Geometry: final body of the model. Coordinates: model frame, mm. Coordinates: 2 decimals unless noted, no trailing zeros. Loops run counter-clockwise (first coordinate to the right, second up) from the corner with the lowest first, then second, coordinate; pieces in that order, holes last. Notation, with made-up numbers: (32, 12.5) - (83, 12.5) arc R24 cw to (83, 41.5) - close; hole circle Ø1 at (8.25, 55). An arc over 180 degrees is marked (long way). Answer in a Markdown table with one row per item.
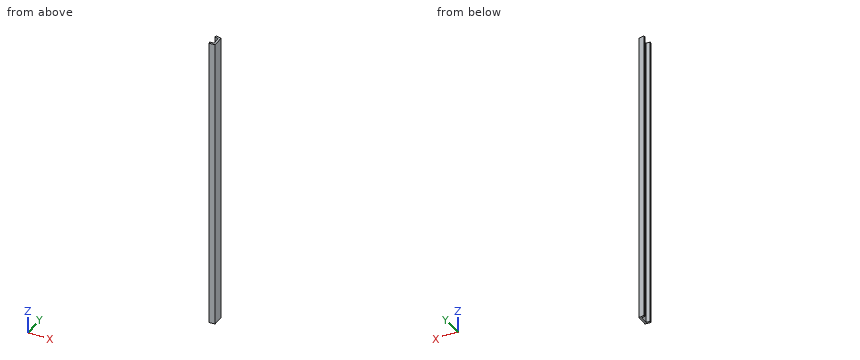
from build123d import *

# Parameters (mm, degrees)
BOSS_EXTRUDE1_DEPTH = 750


with BuildPart() as part:
    # Master sketch-Wing Geometry Master Sketc → Boss-Extrude1 (new body)
    with BuildSketch(Plane.XY):
        with BuildLine():
            Line((224.93, -6.178926254), (224.93, 22.373189537))
            add(Edge.make_bspline(
                [(224.93, 22.373189537), (223.937151031, 22.604229635), (221.53569088, 23.158078559), (217.696277573, 24.019984904), (214.083050592, 24.807059628), (211.880072571, 25.27832033), (211.114806417, 25.441064095)],
                knots=[0.125197771, 0.125197771, 0.125197771, 0.125197771, 0.130088746, 0.137022467, 0.144077656, 0.147831525, 0.147831525, 0.147831525, 0.147831525], degree=3))
            Line((211.114806417, 25.441064095), (210.07475011, 20.55043194))
            Line((210.07475011, 20.55043194), (219.93, 18.391622486))
            Line((219.93, 18.391622486), (219.93, -1.558186688))
            Line((219.93, -1.558186688), (209.78690169, -2.365451127))
            Line((209.78690169, -2.365451127), (210.173597999, -7.350571372))
            add(Edge.make_bspline(
                [(210.173597999, -7.350571372), (210.519069964, -7.323773075), (212.294721257, -7.18589941), (215.480211959, -6.932652125), (219.709739235, -6.590064586), (222.853288837, -6.342418671), (224.586664849, -6.205927526), (224.93, -6.178926254)],
                knots=[0.856037867, 0.856037867, 0.856037867, 0.856037867, 0.857700425, 0.864583105, 0.871370128, 0.878060224, 0.879712638, 0.879712638, 0.879712638, 0.879712638], degree=3))
        make_face()
    extrude(amount=BOSS_EXTRUDE1_DEPTH)


solid = part.part
(1) Ray query, probe 1 along X at (y, z) = (6.5, 228); probe 2 along Y at (x, z) = (211.25, 639); probe 3 along X at (y, z) = (-3, 270.5). Return the intervals inside material, ascending.
Verdict:
| item | result |
|---|---|
| probe 1 | x = 219.93 to 224.93 |
| probe 2 | y = -7.27 to -2.25, 20.29 to 25.41 |
| probe 3 | x = 209.84 to 224.93 |
(2) First-contact query: pin 1 Ø2 at (x, y) = (217, -2.5) entering from -Z; pin 2 Ø2 at (x, z) = (217.5, 367.5) entering from +Y; pin 3 Ø5 at (x, z) = (213, 194) entering from -Y; pin 4 Ø4 at (x, y) = (215, 17) entering from +Z. Flat tips, straight axial feed; report the tip coordinate or a pass-through.
Verdict:
| item | result |
|---|---|
| pin 1 | stops at z = 0 |
| pin 2 | stops at y = 24.28 |
| pin 3 | stops at y = -7.33 |
| pin 4 | passes through |
(3) Cut plane A-A on y = 6. Output: boundary loops of the cut face in (x, z).
Verdict:
| item | result |
|---|---|
| outline | (219.93, 0) - (224.93, 0) - (224.93, 750) - (219.93, 750) - close |
